For this review, take the finished solid that the model builds, in its own axes (mm). Face numbers are marked on the shaded views. A direction names the side the tool comes from. Give positions to 0.01 mm unless a question says otherwise; leave off trailing zeros. Order: outer loops, then holes, each group sorted by start corner. A loop starts at its lowest first (then second) coordinate and runs counter-clockwise, first axis right, second up. Notation, with made-up numbers: M -28.5,28 L 11.5,28 A28 cw 11.5,56 Z; hole C 89.25,32.5 d11. An arc over 180 degrees is marked long. Answer as CSV lines item,"result". Start each with the question number.
1. For line 1 along Y through (x, z) = (25.75, 0); line 2 along Y through (x, z) = (6.5, 0); line 3 along X through (y, z) = (4.8, 0), list the stretches that pass through material, from the lowest coordinate up.
2. We need section C-C, the plane x = 4. Give the boundary of the cut face in (y, z), and give its area (3 significant figures).
3. We need section B-B, the plane y = 0. Give the boundary of the cut face in (x, z).
4. We need section D-D, the plane x = 10.5. Give the boundary of the cut face in (y, z).
5. Clearance check with flat-ended pins moving along their axes: P1, Ø3, axis at x = 20.5, y = -5, coming from the -Z side; P2, Ø1.2, axis at x = 23.5, z = 10.5, coming from the +Y side; P3, Ø10, axis at y = 4.5, z = -4.5, coming from the +X side; P4, Ø6, axis at x = 4, y = -3.5, coming from the +Z side. State where each tip first meets the part, or that it passes through.
6. We need section A-A, the plane z = 0. State how many separate pieces and enclosed holes the cut face has, and give its area (3 significant figures).
7. Mouldability with a two-part tool opening along X and no side actions: class the marked faces 4, 5 and 6 as pulls with the +X half, pulls with the -X half, needs draft (parallel to the pull), parting line crosses it, or undercut.
8. Machinability: for the marked faces 1, 2 and 3, which of the approach directions +Z, -Z, +X, -X, +Y, -Y give a long, thin tool a straight path to every point of the face, cutting with its end or side? Answer none if there is none.
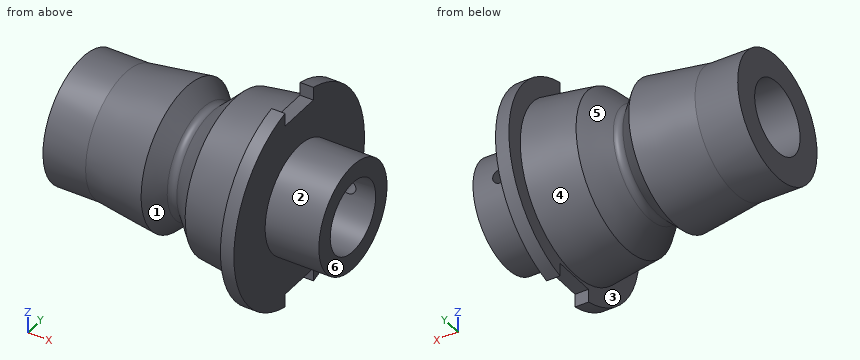
from build123d import *

# Parameters (mm, degrees)
SKETCH3_W                  = 2
SKETCH3_H                  = 5
CUT_EXTRUDE6_DEPTH         = 30.137659458
SKETCH2_R                  = 2.5
CUT_EXTRUDE7_DEPTH         = 30.030211827
SKETCH4_R                  = 6
SKETCH4_R_2                = 4
BOSS_EXTRUDE1_DEPTH        = 6
SKETCH5_R                  = 4
CUT_EXTRUDE8_DEPTH         = 25
M2X0_4_TAPPED_HOLE1_REACH  = 38.645
M2X0_4_TAPPED_HOLE1_BORE_R = 0.8


with BuildPart() as part:
    # Sketch1 → Revolve3 (revolve)
    with BuildSketch(Plane.XY, mode=Mode.PRIVATE) as revolve3_sk:
        with BuildLine():
            Line((0, 0), (0, 6.982))
            Line((0, 6.982), (4.76, 6.982))
            Line((4.76, 6.982), (11.56, 7.937677676))
            Line((11.56, 7.937677676), (13.343138593, 6.154539083))
            ThreePointArc((13.343138593, 6.154539083), (13.880539746, 5.931940237), (14.4179409, 6.154539083))
            Line((14.4179409, 6.154539083), (16.96, 8.696598183))
            Line((16.96, 8.696598183), (22.676500961, 9.5))
            Line((22.676500961, 9.5), (22.676500961, 11.5))
            Line((22.676500961, 11.5), (24.176500961, 11.5))
            Line((24.176500961, 11.5), (24.176500961, 0))
            Line((24.176500961, 0), (0, 0))
        make_face()
    revolve(revolve3_sk.sketch.rotate(Axis((24.176500961, 0, 0), (-1, 0, 0)), 90), axis=Axis((24.176500961, 0, 0), (-1, 0, 0)))

    # Sketch3 → Cut-Extrude6 (cut, through all)
    with BuildSketch(Plane(origin=(24.176500961, 0, 0), x_dir=(0, 0, -1), z_dir=(1, 0, 0))):
        with Locations((-10.75, 0)):
            Rectangle(SKETCH3_W, SKETCH3_H)
        with Locations((10.75, 0)):
            Rectangle(SKETCH3_W, SKETCH3_H)
    extrude(amount=-CUT_EXTRUDE6_DEPTH, mode=Mode.SUBTRACT)

    # Sketch2 → Cut-Extrude7 (cut, through all)
    with BuildSketch(Plane(origin=(0, 0, 0), x_dir=(0, 0, -1), z_dir=(1, 0, 0))):
        Circle(SKETCH2_R)
    extrude(amount=CUT_EXTRUDE7_DEPTH, mode=Mode.SUBTRACT)

    # Sketch4 → Boss-Extrude1 (add)
    with BuildSketch(Plane(origin=(24.176500961, 0, 0), x_dir=(0, 0, -1), z_dir=(1, 0, 0))):
        Circle(SKETCH4_R)
        Circle(SKETCH4_R_2, mode=Mode.SUBTRACT)
    extrude(amount=BOSS_EXTRUDE1_DEPTH)

    # Sketch5 → Cut-Extrude8 (cut)
    with BuildSketch(Plane(origin=(24.176500961, 0, 0), x_dir=(0, 0, -1), z_dir=(1, 0, 0))):
        with Locations(Location((0, 0, 0), (0, 0, 180))):
            Circle(SKETCH5_R)
    extrude(amount=-CUT_EXTRUDE8_DEPTH, mode=Mode.SUBTRACT)

    # M2x0.4 Tapped Hole1 bore → M2x0.4 Tapped Hole1 (cut, up to next)
    with BuildSketch(Plane(origin=(0, 6, 0), x_dir=(1, 0, 0), z_dir=(0, 1, 0)), mode=Mode.PRIVATE) as m2x0_4_tapped_hole1_sk1:
        with Locations((27.176500961, 0)):
            Circle(M2X0_4_TAPPED_HOLE1_BORE_R)
    m2x0_4_tapped_hole1_tool1 = extrude(m2x0_4_tapped_hole1_sk1.sketch, amount=-M2X0_4_TAPPED_HOLE1_REACH, mode=Mode.PRIVATE) & part.part
    add(m2x0_4_tapped_hole1_tool1.solids().sort_by_distance((27.176501, 6, 0))[0], mode=Mode.SUBTRACT)


solid = part.part
Result set:
1,line 1,"-6 to -4, 4 to 6"
1,line 2,"-7.23 to -4, 4 to 7.23"
1,line 3,"0 to 26.38, 27.98 to 30.18"
2,outline,"C 0,0 d13.96; hole C 0,0 d8"
2,area,"103 mm2"
3,outline,"M 0,-6.98 L 4.76,-6.98 L 11.56,-7.94 L 13.34,-6.15 A0.76 cw 14.42,-6.15 L 16.96,-8.7 L 22.68,-9.5 L 22.68,-9.75 L 24.18,-9.75 L 24.18,-6 L 30.18,-6 L 30.18,-4 L 0,-4 Z; M 0,4 L 30.18,4 L 30.18,6 L 24.18,6 L 24.18,9.75 L 22.68,9.75 L 22.68,9.5 L 16.96,8.7 L 14.42,6.15 A0.76 cw 13.34,6.15 L 11.56,7.94 L 4.76,6.98 L 0,6.98 Z"
4,outline,"C 0,0 d15.58; hole C 0,0 d8"
5,P1,"z = -8.54"
5,P2,"y = 5.85"
5,P3,"x = 30.18"
5,P4,"z = 7.04"
6,separate pieces,"3"
6,enclosed holes,"0"
6,area,"210 mm2"
7,face 4,"pulls with the -X half"
7,face 5,"undercut"
7,face 6,"pulls with the +X half"
8,face 1,"none"
8,face 2,"+X"
8,face 3,"-X"
